Verification items for this drawing (mm, ordinates from the low corner). Round coordinates to 2 decimals unless told otherwise and drop trailing zeros. Write each loop counter-clockwise with the first axis right and the second up, starting at its lowest first coordinate (ties: lowest second). Pieces come first, ordered by that corner, then holes.
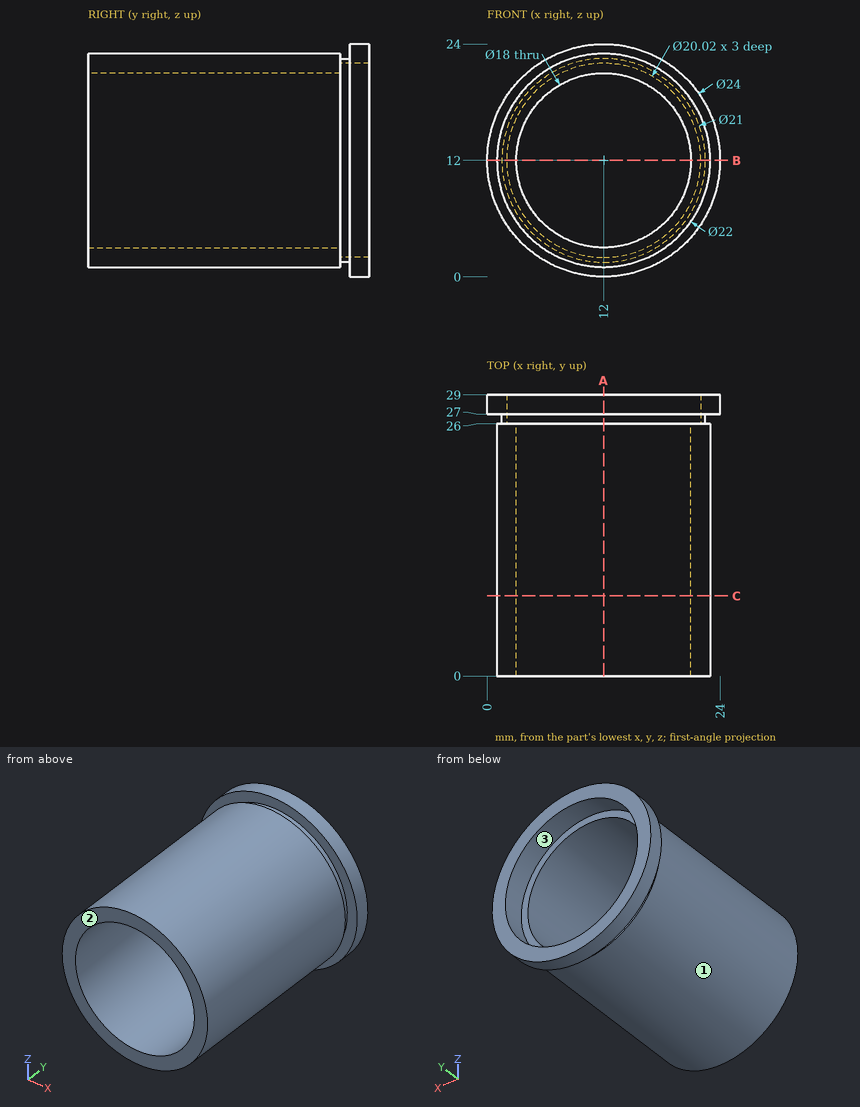
1. Section check B-B (z = 12). Record the cut outline in (x, y).
2. Release check for a two-part mould opening along Z. For the marked faces 1, 2 and 3 record: +Z half, -Z half, draft (parallel to the pull), parting line (faces both ways), or undercut.
3. Scan lines: line 1 along X through (y, z) = (26.9, 12); line 2 along X through (y, z) = (8.25, 12); line 3 along Y through (x, z) = (22.5, 7). Record each from-to range of solid material in increasing order.
4. Section check C-C (y = 8.25). Record the cut outline in (x, z).
5. Section check A-A (x = 12). Record the cut outline in (y, z).
6. Depth check by flat-ended pin: pin 1 Ø6 at (y, z) = (26, 8.5) entering from -X; pin 2 Ø4 at (x, z) = (3, 17) entering from -Y; pin 3 Ø6 at (x, y) = (3, 5.5) entering from +Z; pin 4 Ø1.5 at (x, y) = (4.5, 5) entering from -Z. Enter the tip coordinate at first touch or a pass-through.
Results below:
1. outline: (0, 27) - (1.5, 27) - (1.5, 26) - (1, 26) - (1, 0) - (3, 0) - (3, 26) - (1.99, 26) - (1.99, 29) - (0, 29) - close; (21, 0) - (23, 0) - (23, 26) - (22.5, 26) - (22.5, 27) - (24, 27) - (24, 29) - (22.01, 29) - (22.01, 26) - (21, 26) - close
2. face 1: parting line
2. face 2: draft
2. face 3: undercut
3. line 1: x = 1.5 to 1.99, 22.01 to 22.5
3. line 2: x = 1 to 3, 21 to 23
3. line 3: y = 27 to 29
4. outline: circle Ø22 at (12, 12); hole circle Ø18 at (12, 12)
5. outline: (0, 1) - (26, 1) - (26, 1.5) - (27, 1.5) - (27, 0) - (29, 0) - (29, 1.99) - (26, 1.99) - (26, 3) - (0, 3) - close; (0, 21) - (26, 21) - (26, 22.01) - (29, 22.01) - (29, 24) - (27, 24) - (27, 22.5) - (26, 22.5) - (26, 23) - (0, 23) - close
6. pin 1: stops at x = 0.02
6. pin 2: stops at y = 0
6. pin 3: stops at z = 21.22
6. pin 4: stops at z = 3.31
